Could you check a few things on this model? Use its own coordinates, in mm. A direction names the side the tool comes from. Round coordinates to 2 decimals unless told otherwise and drop trailing zeros. Loops run counter-clockwise (first coordinate to the right, second up) from the corner with the lowest first, then second, coordinate; pieces in that order, holes last.
from build123d import *

# Parameters (mm, degrees)
BOSS_EXTRU_1_DEPTH      = 4
ESQUISSE3_R             = 3.5
ESQUISSE3_R_2           = 1.6
ENL_V_MAT_EXTRU_1_DEPTH = 5
ENL_V_MAT_EXTRU_2_DEPTH = 2
CONG_1_R                = 1


with BuildPart() as part:
    # Esquisse1 → Boss.-Extru.1 (new body)
    with BuildSketch(Plane.XY):
        with BuildLine():
            Line((-27.254178511, 7), (-13.254178511, 7))
            ThreePointArc((-13.254178511, 7), (-6.254178511, 0), (-13.254178511, -7))
            Line((-13.254178511, -7), (-27.254178511, -7))
            ThreePointArc((-27.254178511, -7), (-34.254178511, 0), (-27.254178511, 7))
        make_face()
    extrude(amount=BOSS_EXTRU_1_DEPTH)

    # Esquisse3 → Enlèv. mat.-Extru.1 (cut, through all)
    with BuildSketch(Plane.XY.offset(4)):
        with Locations((-20.254178511, 0)):
            Circle(ESQUISSE3_R)
        with Locations((-30.254178511, 0)):
            Circle(ESQUISSE3_R_2)
        with Locations((-10.254178511, 0)):
            Circle(ESQUISSE3_R_2)
    extrude(amount=-ENL_V_MAT_EXTRU_1_DEPTH, mode=Mode.SUBTRACT)

    # Esquisse4 → Enlèv. mat.-Extru.2 (cut)
    with BuildSketch(Plane.XY.offset(4)):
        Polygon((-22.563579588, 4), (-24.872980665, 0), (-22.563579588, -4), (-17.944777434, -4), (-15.635376357, 0), (-17.944777434, 4), align=None)
    extrude(amount=-ENL_V_MAT_EXTRU_2_DEPTH, mode=Mode.SUBTRACT)

    # Congé1
    cong_1_edges = [part.edges().sort_by_distance(p)[0] for p in [
        (-6.254178511, 0, 4),
        (-20.254178511, 7, 4),
        (-34.254178511, 0, 4),
        (-20.254178511, 7, 0),
        (-6.254178511, 0, 0),
        (-20.254178511, -7, 0),
        (-34.254178511, 0, 0),
        (-20.254178511, -7, 4),
    ]]
    fillet(cong_1_edges, radius=CONG_1_R)


solid = part.part
Item 1: Will these pins go through, and if not, where does the flat tip stop? pin 1 (1.5 mm diameter, centred on x = -30, y = 2, fed in from -Z); pin 2 (2.5 mm diameter, centred on x = -22.5, y = 0.5, fed in from +Z); pin 3 (1.5 mm diameter, centred on y = -2, z = 1.5, fed in from -X); pin 4 (1 mm diameter, centred on y = 5, z = 1.5, fed in from -X).
Results list:
pin 1: stops at z = 0
pin 2: stops at z = 2
pin 3: stops at x = -34.14
pin 4: stops at x = -32.62
Item 2: If we section it at A-A, the plane z = 1.45: Please give me the cut outline in (x, y), then the cut area to 3 significant figures.
Results list:
outline: (-27.25, -7) - (-13.25, -7) arc R7 ccw to (-13.25, 7) - (-27.25, 7) arc R7 ccw to start; hole circle Ø3.2 at (-30.25, 0); hole circle Ø7 at (-20.25, 0); hole circle Ø3.2 at (-10.25, 0)
area: 295 mm2
Item 3: For faces 1 (the cylindrical face through (-16.916, 1.051, 1.014)), 2 (the flat face through (-17, 2, 2)), which set-ups out of +Z, -Z, +X, -X, +Y, -Y let a thin tool reach every point of the face, with its end or its side?
Results list:
face 1: +Z, -Z
face 2: +Z
Item 4: If we section it at C-C, the plane x = -25.25: Please give me the cut outline in (y, z), then the cut area to 3 significant figures.
Results list:
outline: (-7, 1) arc R1 ccw to (-6, 0) - (6, 0) arc R1 ccw to (7, 1) - (7, 3) arc R1 ccw to (6, 4) - (-6, 4) arc R1 ccw to (-7, 3) - close
area: 55.1 mm2
Item 5: If I drill on line 1 along X through (y, z) = (0.5, 0.45); line 2 along X through (y, z) = (0.75, 0.3); line 3 along X through (y, z) = (-3.5, 3.2), over which ranges is the centre line in solid material (lowest first)?
Results list:
line 1: x = -34.07 to -31.77, -28.73 to -23.72, -16.79 to -11.77, -8.73 to -6.44
line 2: x = -33.93 to -31.67, -28.84 to -23.67, -16.84 to -11.67, -8.84 to -6.58
line 3: x = -33.29 to -22.85, -17.66 to -7.22
Item 6: We'd pull the mould along Y, two halves only. Please class faces 3 (the flat face through (-20, -7, 2)), 4 (the flat face through (-17, 3, 4)), 5 (the flat face through (-20, 4, 3)), 6 (the cylindrical face through (-28.728, 0.481, 2.028)): released by +Y, released by -Y, zero draft, split by the parting line, or undercut.
Results list:
face 3: released by -Y
face 4: zero draft
face 5: undercut
face 6: undercut
Item 7: If we section it at B-B, the plane x = -20.75: Please give me the cut outline in (y, z).
Results list:
outline: (-7, 1) arc R1 ccw to (-6, 0) - (-3.46, 0) - (-3.46, 2) - (-4, 2) - (-4, 4) - (-6, 4) arc R1 ccw to (-7, 3) - close; (3.46, 0) - (6, 0) arc R1 ccw to (7, 1) - (7, 3) arc R1 ccw to (6, 4) - (4, 4) - (4, 2) - (3.46, 2) - close
